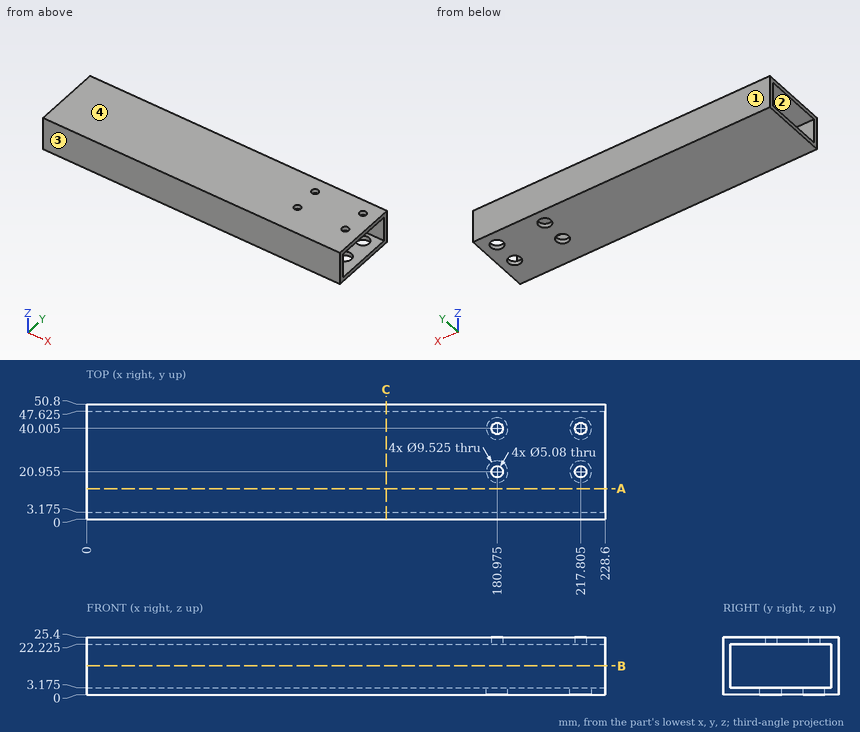
Print and shaded views of the part. All mm, measured from the part's lowest x, y and z. Round coordinates to 2 decimals unless told otherwise and drop trailing zeros. Order: outer loops, then holes, each group sorted by start corner. A loop starts at its lowest first (then second) coordinate and runs counter-clockwise, first axis right, second up. Notation, with made-up numbers: (21, -33) - (49, -33) arc R7 cw to (49, -26) - close; hole circle Ø8 at (-35, -3). An arc over 180 degrees is marked (long way). Use a Markdown table: item, result.
1) Pull direction Y, two halves, no side cores. Call the marked faces 1, 2, 3 and 4: pulls with the +Y half, pulls with the -Y half, needs draft (parallel to the pull), parting line crosses it, or undercut.
Recorded:
| item | result |
|---|---|
| face 1 | pulls with the +Y half |
| face 2 | undercut |
| face 3 | pulls with the -Y half |
| face 4 | needs draft |
2) Wall check: L1, parallel to Y at x = 156, z = 4.75 (3 decimals); L2, parallel to Z at x = 42, y = 31.5 (3 decimals). Give the ranges that are in metal, low to high.
Recorded:
| item | result |
|---|---|
| L1 | y = 0 to 3.175, 47.625 to 50.8 |
| L2 | z = 0 to 3.175, 22.225 to 25.4 |
3) Saw through at A-A on y = 13.5. Write the cut outline in (x, z) (3 decimals).
Recorded:
| item | result |
|---|---|
| outline | (0, 0) - (228.6, 0) - (228.6, 3.175) - (0, 3.175) - close; (0, 22.225) - (228.6, 22.225) - (228.6, 25.4) - (0, 25.4) - close |
4) Saw through at C-C on x = 132. Write the cut outline in (y, z) (3 decimals).
Recorded:
| item | result |
|---|---|
| outline | (0, 0) - (50.8, 0) - (50.8, 25.4) - (0, 25.4) - close; hole (3.175, 3.175) - (47.625, 3.175) - (47.625, 22.225) - (3.175, 22.225) - close |
5) Flat gauge pins, fed straight in: pin 1 Ø1 at (y, z) = (29.5, 21.5) entering from -X; pin 2 Ø5.5 at (x, y) = (180.975, 40.005) entering from -Z (3 decimals). Where does each tip first touch, or does it go through?
Recorded:
| item | result |
|---|---|
| pin 1 | passes through |
| pin 2 | stops at z = 22.225 |
6) Saw through at B-B on z = 12.75. Write the cut outline in (x, y) (3 decimals).
Recorded:
| item | result |
|---|---|
| outline | (0, 0) - (228.6, 0) - (228.6, 3.175) - (0, 3.175) - close; (0, 47.625) - (228.6, 47.625) - (228.6, 50.8) - (0, 50.8) - close |
